Source: CAD feature listing. Evaluate the final solid. Frame: model axes, mm. Face numbers are marked on the shaded views. A direction names the side the tool comes from. Round coordinates to 2 decimals unless told otherwise and drop trailing zeros. Loops run counter-clockwise (first coordinate to the right, second up) from the corner with the lowest first, then second, coordinate; pieces in that order, holes last.
Item 1: Section query A-A on x = 0. Return loops of the section in (y, z).
Item 2: Section query B-B on z = 0. Return loops of the section in (x, y).
Item 3: Section query C-C on y = 1.75. Return loops of the section in (x, z), then the cut area to 3 significant figures.
Item 4: Section query D-D on y = 0.7. Return loops of the section in (x, z), then the cut area to 3 significant figures.
Item 5: Access query for the marked faces 1 and 2. Directions: +Z, -Z, +X, -X, +Y, -Y. A direction counts if a zero-diameter tool reaches every point of the face in a straight line with its end or side. Return the directions, or none.
Item 6: Ray query, L1, parallel to Z at x = 0, y = 2; L2, parallel to X at y = 1.05, z = 0. Return the intervals inside material, ascending.
```python
from build123d import *

# Parameters (mm, degrees)
SKETCH1_R           = 2.78
BOSS_EXTRUDE1_DEPTH = 1.5
CHAMFER1_SIZE       = 0.2
SKETCH2_R           = 2.34
BOSS_EXTRUDE2_DEPTH = 1.53
CHAMFER2_SIZE       = 0.2
SKETCH3_R           = 1.6
CUT_EXTRUDE1_DEPTH  = 4.03


with BuildPart() as part:
    # Sketch1 → Boss-Extrude1 (new body)
    with BuildSketch(Plane(origin=(0, 0, 0), x_dir=(1, 0, 0), z_dir=(0, 1, 0))):
        Circle(SKETCH1_R)
    extrude(amount=BOSS_EXTRUDE1_DEPTH)

    # Chamfer1
    chamfer1_edges = [part.edges().sort_by_distance(p)[0] for p in [
        (-2.78, 0, 0),
        (-2.78, 1.5, 0),
    ]]
    chamfer(chamfer1_edges, length=CHAMFER1_SIZE)

    # Sketch2 → Boss-Extrude2 (add)
    with BuildSketch(Plane(origin=(0, 1.5, 0), x_dir=(1, 0, 0), z_dir=(0, 1, 0))):
        Circle(SKETCH2_R)
    extrude(amount=BOSS_EXTRUDE2_DEPTH)

    # Chamfer2
    chamfer2_edges = [part.edges().sort_by_distance(p)[0] for p in [
        (-2.34, 3.03, 0),
    ]]
    chamfer(chamfer2_edges, length=CHAMFER2_SIZE)

    # Sketch3 → Cut-Extrude1 (cut, through all)
    with BuildSketch(Plane(origin=(0, 3.03, 0), x_dir=(1, 0, 0), z_dir=(0, 1, 0))):
        Circle(SKETCH3_R)
    extrude(amount=-CUT_EXTRUDE1_DEPTH, mode=Mode.SUBTRACT)


solid = part.part
```
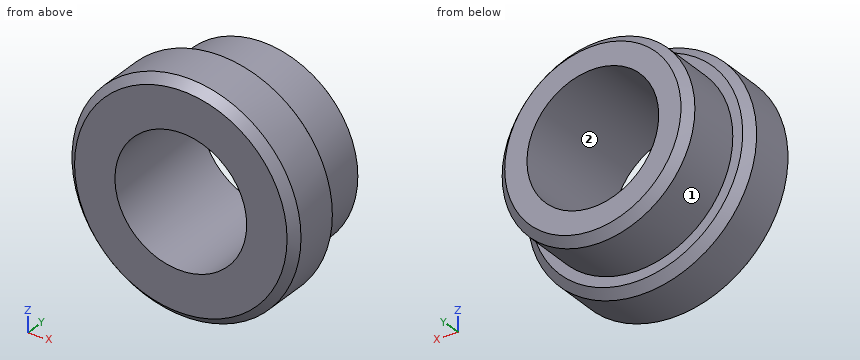
Data:
1. outline: (0, -2.58) - (0.2, -2.78) - (1.3, -2.78) - (1.5, -2.58) - (1.5, -2.34) - (2.83, -2.34) - (3.03, -2.14) - (3.03, -1.6) - (0, -1.6) - close; (0, 1.6) - (3.03, 1.6) - (3.03, 2.14) - (2.83, 2.34) - (1.5, 2.34) - (1.5, 2.58) - (1.3, 2.78) - (0.2, 2.78) - (0, 2.58) - close
2. outline: (-2.78, 0.2) - (-2.58, 0) - (-1.6, 0) - (-1.6, 3.03) - (-2.14, 3.03) - (-2.34, 2.83) - (-2.34, 1.5) - (-2.58, 1.5) - (-2.78, 1.3) - close; (1.6, 0) - (2.58, 0) - (2.78, 0.2) - (2.78, 1.3) - (2.58, 1.5) - (2.34, 1.5) - (2.34, 2.83) - (2.14, 3.03) - (1.6, 3.03) - close
3. outline: circle Ø4.68 at (0, 0); hole circle Ø3.2 at (0, 0)
3. area: 9.16 mm2
4. outline: circle Ø5.56 at (0, 0); hole circle Ø3.2 at (0, 0)
4. area: 16.2 mm2
5. face 1: +Y
5. face 2: +Y, -Y
6. L1: z = -2.34 to -1.6, 1.6 to 2.34
6. L2: x = -2.78 to -1.6, 1.6 to 2.78
